Geometry: final body of the model. Coordinates: model frame, mm. A direction names the side the tool comes from. Coordinates: 2 decimals unless noted, no trailing zeros. Write each loop counter-clockwise with the first axis right and the second up, starting at its lowest first coordinate (ties: lowest second). Pieces come first, ordered by that corner, then holes. Notation, with made-up numbers: (48, 64.5) - (55, 64.5) arc R12 cw to (55, 75.5) - close; hole circle Ø6 at (-9.75, 4). An arc over 180 degrees is marked (long way). Put each result on its own line as item: value.
```python
from build123d import *

# Parameters (mm, degrees)
BOSS_EXTRUDE1_DEPTH = 2
SKETCH2_R           = 2
BOSS_EXTRUDE2_DEPTH = 6.7
CHAMFER1_SIZE       = 0.5
FILLET1_R           = 0.2


with BuildPart() as part:
    # Sketch1 → Boss-Extrude1 (new body)
    with BuildSketch(Plane(origin=(0, 0, 0), x_dir=(1, 0, 0), z_dir=(0, 1, 0))):
        Polygon((0, 2.886751346), (-2.5, 1.443375673), (-2.5, -1.443375673), (0, -2.886751346), (2.5, -1.443375673), (2.5, 1.443375673), align=None)
    extrude(amount=BOSS_EXTRUDE1_DEPTH)

    # Sketch2 → Boss-Extrude2 (add)
    with BuildSketch(Plane(origin=(0, 2, 0), x_dir=(1, 0, 0), z_dir=(0, 1, 0))):
        Circle(SKETCH2_R)
    extrude(amount=BOSS_EXTRUDE2_DEPTH)

    # Chamfer1
    chamfer1_edges = [part.edges().sort_by_distance(p)[0] for p in [
        (-2, 8.7, 0),
    ]]
    chamfer(chamfer1_edges, length=CHAMFER1_SIZE)

    # Fillet1
    fillet1_edges = [part.edges().sort_by_distance(p)[0] for p in [
        (-2, 2, 0),
    ]]
    fillet(fillet1_edges, radius=FILLET1_R)


solid = part.part
```
1. Section query B-B (y = 1.75). Return loops of the section in (x, z), then the cut area to 3 significant figures.
Answer below:
outline: (-2.5, -1.44) - (0, -2.89) - (2.5, -1.44) - (2.5, 1.44) - (0, 2.89) - (-2.5, 1.44) - close
area: 21.7 mm²
2. Section query C-C (y = 5). Return loops of the section in (x, z), then the cut area to 3 significant figures.
Answer below:
outline: circle Ø4 at (0, 0)
area: 12.6 mm²
3. Section query A-A (z = 0). Return loops of the section in (x, y).
Answer below:
outline: (-2.5, 0) - (2.5, 0) - (2.5, 2) - (2.2, 2) arc R0.2 cw to (2, 2.2) - (2, 8.2) - (1.5, 8.7) - (-1.5, 8.7) - (-2, 8.2) - (-2, 2.2) arc R0.2 cw to (-2.2, 2) - (-2.5, 2) - close
4. Section query D-D (z = -2.5). Return loops of the section in (x, y), then the cut area to 3 significant figures.
Answer below:
outline: (-0.67, 0) - (0.67, 0) - (0.67, 2) - (-0.67, 2) - close
area: 2.68 mm²
5. Set-up query: faces 1 (the cylindrical face through (0, 5, 2)), 2 (the flat face through (1.267, 0.986, -2.155)). Return all of +Z, -Z, +X, -X, +Y, -Y with unobstructed straight access to the full face (end or side cutting, diameter ignored); none if empty.
Answer below:
face 1: +Y
face 2: -Z, +X, +Y, -Y
6. Ray query, probe 1 along Y at (x, z) = (-0.9, 2.25); probe 2 along X at (y, z) = (8, 0.2); probe 3 along X at (y, z) = (0.5, -1.65). Return the intervals inside material, ascending. Write a range as from..to.
Answer below:
probe 1: y = 0..2
probe 2: x = -1.99..1.99
probe 3: x = -2.14..2.14
7. Pin query (flat end, axial travel): pin 1 Ø3 at (y, z) = (5.5, -0.5) entering from -X; pin 2 Ø1 at (y, z) = (4.5, 1.5) entering from -X; pin 3 Ø3 at (x, z) = (-1.5, 1) entering from -Y. Return the tip coordinate at first contact, or that it passes through.
Answer below:
pin 1: stops at x = -2
pin 2: stops at x = -1.73
pin 3: stops at y = 0
